```python
from build123d import *

# Parameters (mm, degrees)
SKETCH1_W           = 25.4
SKETCH1_H           = 20
SKETCH1_R           = 2.75
BOSS_EXTRUDE1_DEPTH = 3
SKETCH2_W           = 25.4
SKETCH2_H           = 25.75
SKETCH2_R           = 1.3
BOSS_EXTRUDE2_DEPTH = 5
FILLET1_R           = 1
FILLET2_R           = 1


with BuildPart() as part:
    # Sketch1 → Boss-Extrude1 (new body)
    with BuildSketch(Plane.XY):
        Rectangle(SKETCH1_W, SKETCH1_H)
        with Locations((6.7, 0)):
            Circle(SKETCH1_R, mode=Mode.SUBTRACT)
        with Locations(Location((-6.7, 0, 0), (0, 0, 180))):
            Circle(SKETCH1_R, mode=Mode.SUBTRACT)
    extrude(amount=BOSS_EXTRUDE1_DEPTH)

    # Sketch2 → Boss-Extrude2 (add)
    with BuildSketch(Plane.XY):
        with Locations((0, -19.875)):
            Rectangle(SKETCH2_W, SKETCH2_H)
        with Locations((-3.5, -19)):
            Circle(SKETCH2_R, mode=Mode.SUBTRACT)
        with Locations((3.5, -13.5)):
            Circle(SKETCH2_R, mode=Mode.SUBTRACT)
        with BuildLine():
            Line((-7.426009093, -23), (7.426009093, -23))
            ThreePointArc((7.426009093, -23), (8.426009093, -24), (7.426009093, -25))
            Line((7.426009093, -25), (-7.426009093, -25))
            ThreePointArc((-7.426009093, -25), (-8.426009093, -24), (-7.426009093, -23))
        make_face(mode=Mode.SUBTRACT)
        with BuildLine():
            Line((-7.426009093, -29.880803462), (7.426009093, -29.880803462))
            ThreePointArc((7.426009093, -29.880803462), (8.426009093, -28.880803462), (7.426009093, -27.880803462))
            Line((7.426009093, -27.880803462), (-7.426009093, -27.880803462))
            ThreePointArc((-7.426009093, -27.880803462), (-8.426009093, -28.880803462), (-7.426009093, -29.880803462))
        make_face(mode=Mode.SUBTRACT)
    extrude(amount=BOSS_EXTRUDE2_DEPTH)

    # Fillet1
    fillet1_edges = [part.edges().sort_by_distance(p)[0] for p in [
        (-8.426009093, -24, 0),
        (0, -25, 0),
        (8.426009093, -24, 0),
        (0, -23, 0),
        (-8.426009093, -28.880803462, 0),
        (0, -29.880803462, 0),
        (8.426009093, -28.880803462, 0),
        (0, -27.880803462, 0),
    ]]
    fillet(fillet1_edges, radius=FILLET1_R)

    # Fillet2
    fillet2_edges = [part.edges().sort_by_distance(p)[0] for p in [
        (0, 10, 3),
        (0, -7, 5),
        (0, -7, 3),
        (12.7, -32.75, 2.5),
        (-12.7, -32.75, 2.5),
    ]]
    fillet(fillet2_edges, radius=FILLET2_R - 0.0001)  # a hair under: the kernel refuses the full size


solid = part.part
```
Geometry: final body of the model. Coordinates: model frame, mm. A direction names the side the tool comes from. Coordinates: 2 decimals unless noted, no trailing zeros. Write each loop counter-clockwise with the first axis right and the second up, starting at its lowest first coordinate (ties: lowest second). Pieces come first, ordered by that corner, then holes. Notation, with made-up numbers: M 31,-34 L 64,-34 A6 cw 64,-28 Z; hole C 3,76 d7. An arc over 180 degrees is marked long. Use CSV: the item, a comma, the result in double quotes. Start each with the question number.
1. Cut plane C-C on z = 1.55. Return the cut outline in (x, y).
2. First-contact query: P1, Ø4.5, axis at x = 3.5, y = 0, coming from the +Z side. Flat tip, straight axial feed; report the tip coordinate or a pass-through.
3. Cut plane B-B on x = 6.7. Count the separate pieces of the cut face and the enclosed holes in it, plus the area to 3 significant figures.
4. Reachability of faces 5 (the face through (12.7, -16, 2)), 6 (the face through (0, -23, 3)), 7 (the face through (0.104, -22.699, 0.285)), 8 (the face through (0, 2, 3)) from +Z, -Z, +X, -X, +Y, -Y: full face, straight path, thin tool, end or side. Return the list, or none.
5. Ray query, probe 1 along Y at (x, z) = (1, 3.9) (3 decimals); probe 2 along Y at (x, z) = (-3.5, 1.6); probe 3 along Y at (x, z) = (6.7, 1.65). Return the intervals inside material, ascending.
6. Cut plane A-A on y = 0. Return the cut outline in (x, z), plus the area to 3 significant figures.
7. Cut plane D-D on y = -19. Return the cut outline in (x, z).
8. Mould query, pull axis X, two halves, no side actions, for faces 1 (the face through (0, -20, 5)), 2 (the face through (-12.7, -16, 2)), 3 (the face through (12.399, -32.465, 2.535)), 4 (the face through (-0.104, -25.301, 0.285)). Classes: pulls with the +X half, pulls with the -X half, needs draft (parallel to the pull), parting line crosses it, or undercut.
Entries:
1,outline,"M -12.7,-31.75 A1 ccw -11.7,-32.75 L 11.7,-32.75 A1 ccw 12.7,-31.75 L 12.7,10 L -12.7,10 Z; hole C -6.7,0 d5.5; hole M -7.43,-29.88 L 7.43,-29.88 A1 ccw 7.43,-27.88 L -7.43,-27.88 A1 ccw Z; hole M -7.43,-25 L 7.43,-25 A1 ccw 7.43,-23 L -7.43,-23 A1 ccw Z; hole C -3.5,-19 d2.6; hole C 3.5,-13.5 d2.6; hole C 6.7,0 d5.5"
2,P1,"z = 3"
3,separate pieces,"4"
3,enclosed holes,"0"
3,area,"142 mm²"
4,face 5,"+Z, -Z, +X, +Y, -Y"
4,face 6,"+Z, -Z"
4,face 7,"-Z"
4,face 8,"+Z, +X, -X, +Y"
5,probe 1,"-32.75 to -29.881, -27.881 to -25, -23 to -6.995"
5,probe 2,"-32.75 to -29.88, -27.88 to -25, -23 to -20.3, -17.7 to 10"
5,probe 3,"-32.75 to -29.88, -27.88 to -25, -23 to -2.75, 2.75 to 10"
6,outline,"M -12.7,0 L -9.45,0 L -9.45,3 L -12.7,3 Z; M -3.95,0 L 3.95,0 L 3.95,3 L -3.95,3 Z; M 9.45,0 L 12.7,0 L 12.7,3 L 9.45,3 Z"
6,area,"43.2 mm²"
7,outline,"M -12.7,0 L -4.8,0 L -4.8,5 L -12.7,5 Z; M -2.2,0 L 12.7,0 L 12.7,5 L -2.2,5 Z"
8,face 1,"needs draft"
8,face 2,"pulls with the -X half"
8,face 3,"pulls with the +X half"
8,face 4,"undercut"
